Design review of the part built by this model. Coordinates are the model's own, in mm. A direction names the side the tool comes from. Coordinates: 2 decimals unless noted, no trailing zeros. Write each loop counter-clockwise with the first axis right and the second up, starting at its lowest first coordinate (ties: lowest second). Pieces come first, ordered by that corner, then holes. Notation, with made-up numbers: M -38,27 L -23,27 A25 cw -23,44 Z; hole C 35.25,-1.75 d8. An arc over 180 degrees is marked long. Return JSON: item names as keys, results as strings. Group by question number.
Autodesk Inventor part; units mm, degrees
ref_plane "YZ Plane" through (0, 0, 0) normal (1, 0, 0) x (0, 1, 0)
ref_plane "XZ Plane" through (0, 0, 0) normal (0, 1, 0) x (-1, 0, 0)
ref_plane "XY Plane" through (0, 0, 0) normal (0, 0, 1) x (1, 0, 0)
sketch "Boceto1" plane through (0, 0, 0) normal (0, 1, 0) x (-1, 0, 0)
  circle A0 centre (0, 0) radius 10
  dimension "d3" = 20
extrude "Extrusión1" add sketch "Boceto1" along normal blind 6
sketch "Boceto2" plane through (0, 6, 0) normal (0, 1, 0) x (1, 0, 0)
  circle A0 centre (0, 0) radius 20
  dimension "d6" = 40
extrude "Extrusión2" add sketch "Boceto2" along normal blind 6
sketch "Boceto3" plane through (0, 12, 0) normal (0, 1, 0) x (1, 0, 0)
  circle A0 centre (0, 0) radius 15
  dimension "d9" = 30
extrude "Extrusión3" add sketch "Boceto3" along normal blind 6
sketch "Boceto4" plane through (0, 18, 0) normal (0, 1, 0) x (1, 0, 0)
  circle A0 centre (0, 0) radius 4
  circle A1 centre (0, 0) radius 20
  line L0 (-4, 0) -> (-4, -19.5959)
  line L1 (4, 0) -> (4, -19.5959)
  dimension "d12" = 8
extrude "Extrusión4" cut sketch "Boceto4" against normal through all contours A0 | L1 A1 L0 A0 picked at (0.1607, -14.6269)
sketch "Boceto5" plane through (0, 18, 0) normal (0, 1, 0) x (1, 0, 0)
  circle A0 centre (0, 0) radius 12.5
  dimension "d15" = 25
extrude "Extrusión5" cut sketch "Boceto5" against normal blind 10
sketch "Boceto6" plane through (0, 0, 0) normal (0, -1, 0) x (1, 0, 0)
  circle A0 centre (0, 0) radius 8
  dimension "d18" = 16
extrude "Extrusión6" cut sketch "Boceto6" against normal up to surface (6 mm away)
properties part number "shocks_end" material "Goma"
Item 1: The part is to be moulded in two halves that separate along X. For faces 5 (the cylindrical face through (0, 7, -4)), 6 (the cylindrical face through (-0.823, 8.958, -19.983)), 7 (the flat face through (0, 0, -8.2)), 8 (the flat face through (-4, 9, 12)), say which applies: pulls with the +X half, pulls with the -X half, needs draft (parallel to the pull), parting line crosses it, or undercut.
Item 2: For pin 1 (10 mm diameter, centred on y = 9, z = -8, fed in from -X); pin 2 (1.5 mm diameter, centred on y = 13, z = 9, fed in from +X); pin 3 (1.5 mm diameter, centred on x = -10, y = 7, fed in from -Z), all flat-tipped, find the tip position at first contact; note any pin that passes through.
Item 3: Add section D-D (y = 10). Write out the cut boundary in (x, z).
Item 4: Add section C-C (z = -13.5). Write out the cut boundary in (x, y), plus the area to 3 significant figures.
Item 5: Add section A-A (z = 4). Write out the cut boundary in (x, y), plus the area to 3 significant figures.
Item 6: Add section B-B (x = 0). Write out the cut boundary in (y, z), plus the area to 3 significant figures.
Item 7: For line 1 (X direction, y = 3.65, z = 0); line 2 (X direction, y = 13.75, z = 0); line 3 (Y direction, x = 17, z = 4), list the stretches that pass through material, from the lowest coordinate up.
Item 8: Machinability: for faces 1 (the flat face through (-8, 18, -10)), 2 (the flat face through (3, 8, -3)), 3 (the cylindrical face through (0, 3, -10)), 4 (the flat face through (4, 9, 12)), which of the approach directions +Z, -Z, +X, -X, +Y, -Y give a long, thin tool a straight path to every point of the face, cutting with its end or side? Answer none if there is none.
Geometry check:
{
 "1": {"face 5": "undercut", "face 6": "parting line crosses it", "face 7": "needs draft", "face 8": "undercut"},
 "2": {"pin 1": "x = -19.77", "pin 2": "x = 12.53", "pin 3": "z = -17.73"},
 "3": {"outline": "M -4,11.84 L -4,19.6 A20 ccw long 4,19.6 L 4,11.84 A12.5 cw long Z"},
 "4": {"outline": "M -14.76,6 L 14.76,6 L 14.76,12 L 6.54,12 L 6.54,18 L -6.54,18 L -6.54,12 L -14.76,12 Z", "area": "256 mm^2"},
 "5": {"outline": "M -19.6,6 L -9.17,6 L -9.17,0 L -6.93,0 L -6.93,6 L -4,6 L -4,8 L -11.84,8 L -11.84,18 L -14.46,18 L -14.46,12 L -19.6,12 Z; M 4,6 L 6.93,6 L 6.93,0 L 9.17,0 L 9.17,6 L 19.6,6 L 19.6,12 L 14.46,12 L 14.46,18 L 11.84,18 L 11.84,8 L 4,8 Z", "area": "183 mm^2"},
 "6": {"outline": "M 0,-10 L 6,-10 L 6,-20 L 12,-20 L 12,-15 L 18,-15 L 18,-12.5 L 8,-12.5 L 8,-4 L 6,-4 L 6,-8 L 0,-8 Z", "area": "89.0 mm^2"},
 "7": {"line 1": "-10 to -8, 8 to 10", "line 2": "-15 to -12.5, 12.5 to 15", "line 3": "6 to 12"},
 "8": {"face 1": "+Z, -Z, +X, -X, +Y", "face 2": "+Y", "face 3": "-Y", "face 4": "+Z, +Y, -Y"}
}
